Geometry check sheet. Reference: the model listing, model coordinates, mm. Give positions to 0.01 mm unless a question says otherwise; leave off trailing zeros. Loops run counter-clockwise (first coordinate to the right, second up) from the corner with the lowest first, then second, coordinate; pieces in that order, holes last.
1. Material ranges on L1, parallel to Y at x = 0, z = 31 (3 decimals); L2, parallel to X at y = -5.75, z = 11; L3, parallel to Z at x = 4.25, y = 7.5, recorded low to high.
2. Cross-section at A-A, the plane x = 0. Record the cut outline in (y, z) (3 decimals), plus the area to 3 significant figures.
3. Cross-section at D-D, the plane z = 23. Record the cut outline in (x, y) (3 decimals), plus the area to 3 significant figures.
4. Go/stop test with flat-tipped pins: pin 1 Ø1 at (x, z) = (3.5, 12) entering from +Y; pin 2 Ø3 at (y, z) = (7, 17.5) entering from -X; pin 3 Ø1.5 at (y, z) = (-2, 9.5) entering from +X. Record where each tip stops, or that it passes through.
5. Cross-section at C-C, the plane z = 30. Record the cut outline in (x, y) (3 decimals).
6. Release check for a two-part mould opening along X. For faces 1 (the flat face through (4, 0, 25.4)), 2 (the cylindrical face through (-0.69, -3.1, 31.66)), 3 (the cylindrical face through (-5.12, 4.69, 9.53)), 4 (the conical face through (-3, 0.95, 21.08)) record: +X half, -X half, draft (parallel to the pull), parting line (faces both ways), or undercut.
from build123d import *

# Parameters (mm, degrees)
SKETCH1_R                            = 9.525
BOSS_EXTRUDE1_DEPTH                  = 25.4
SKETCH2_R                            = 3.175
BOSS_EXTRUDE2_DEPTH                  = 12.7
F_1_0_228_DIAMETER_HOLE1_D           = 5.7912
F_35_64_0_54688_DIAMETER_HOLE1_D     = 13.890752
F_35_64_0_54688_DIAMETER_HOLE1_DEPTH = 18.796
F_35_64_0_54688_DIAMETER_HOLE1_TIP   = 4.173202923


with BuildPart() as part:
    # Sketch1 → Boss-Extrude1 (new body)
    with BuildSketch(Plane.XY):
        Circle(SKETCH1_R)
    extrude(amount=BOSS_EXTRUDE1_DEPTH)

    # Sketch2 → Boss-Extrude2 (add)
    with BuildSketch(Plane.XY.offset(25.4)):
        Circle(SKETCH2_R)
    extrude(amount=BOSS_EXTRUDE2_DEPTH)

    # #1 (0.228) Diameter Hole1 (through all)
    with Locations(Plane(origin=(0, 0, 0), x_dir=(-1, 0, 0), z_dir=(0, 0, -1))):
        with Locations((0, 0)):
            Hole(F_1_0_228_DIAMETER_HOLE1_D / 2)

    # 35/64 (0.54688) Diameter Hole1
    with Locations(Plane(origin=(0, 0, 0), x_dir=(-1, 0, 0), z_dir=(0, 0, -1))):
        with Locations((0, 0)):
            Hole(F_35_64_0_54688_DIAMETER_HOLE1_D / 2, depth=F_35_64_0_54688_DIAMETER_HOLE1_DEPTH)
            with Locations((0, 0, -(F_35_64_0_54688_DIAMETER_HOLE1_DEPTH + F_35_64_0_54688_DIAMETER_HOLE1_TIP / 2))):  # 118° drill point
                Cone(0, F_35_64_0_54688_DIAMETER_HOLE1_D / 2, F_35_64_0_54688_DIAMETER_HOLE1_TIP, mode=Mode.SUBTRACT)


solid = part.part
Result:
1. L1: y = -3.175 to -2.896, 2.896 to 3.175
1. L2: x = -7.59 to -3.9, 3.9 to 7.59
1. L3: z = 0 to 25.4
2. outline: (-9.525, 0) - (-6.945, 0) - (-6.945, 18.796) - (-2.896, 21.229) - (-2.896, 38.1) - (-3.175, 38.1) - (-3.175, 25.4) - (-9.525, 25.4) - close; (2.896, 21.229) - (6.945, 18.796) - (6.945, 0) - (9.525, 0) - (9.525, 25.4) - (3.175, 25.4) - (3.175, 38.1) - (2.896, 38.1) - close
2. area: 182 mm2
3. outline: circle Ø19.05 at (0, 0); hole circle Ø5.791 at (0, 0)
3. area: 259 mm2
4. pin 1: stops at y = 9.04
4. pin 2: stops at x = -7.78
4. pin 3: stops at x = 9.44
5. outline: circle Ø6.35 at (0, 0); hole circle Ø5.791 at (0, 0)
6. face 1: draft
6. face 2: parting line
6. face 3: undercut
6. face 4: undercut
